```python
from build123d import *

# Parameters (mm, degrees)
EXTRUDE006_DEPTH = 2
EXTRUDE005_DEPTH = 2.25


with BuildPart() as extrude006:
    # Sketch006 → Extrude006 (new body)
    with BuildSketch(Plane.XZ):
        with BuildLine():
            ThreePointArc((16.9, 15.75), (15.9, 14.75), (16.9, 13.75))
            Line((16.9, 13.75), (23.5, 13.75))
            ThreePointArc((23.5, 13.75), (24.5, 14.75), (23.5, 15.75))
            Line((23.5, 15.75), (16.9, 15.75))
        make_face()
    extrude(amount=EXTRUDE006_DEPTH)


with BuildPart() as extrude006_1:
    # Extrude006 placement: moved
    add(extrude006.part.moved(Location((0, 4, 0))))


with BuildPart() as obj1:
    # Sketch005 → Extrude005 (new body)
    with BuildSketch(Plane.XZ):
        with BuildLine():
            ThreePointArc((16.9, 17.35), (15.9, 16.35), (16.9, 15.35))
            Line((16.9, 15.35), (23.5, 15.35))
            ThreePointArc((23.5, 15.35), (24.5, 16.35), (23.5, 17.35))
            Line((23.5, 17.35), (16.9, 17.35))
        make_face()
    extrude(amount=EXTRUDE005_DEPTH)


with BuildPart() as obj1_1:
    # Extrude005 placement: moved
    add(obj1.part.moved(Location((0, 2, 0))))

    # Fusion008: union Extrude006
    add(extrude006_1.part)


with BuildPart() as obj1_2:
    # Fusion008 placement: moved
    add(obj1_1.part.moved(Location((0, 0.25, 0))))


solid = obj1_2.part
```
For this review, take the finished solid that the model builds, in its own axes (mm). A direction names the side the tool comes from. Coordinates: 2 decimals unless noted, no trailing zeros. Write each loop counter-clockwise with the first axis right and the second up, starting at its lowest first coordinate (ties: lowest second). Pieces come first, ordered by that corner, then holes.
(1) For pin 1 Ø1 at (x, y) = (19.5, 3.5) entering from +Z; pin 2 Ø2 at (y, z) = (1, 15) entering from +X; pin 3 Ø1.1 at (x, y) = (21.5, 1) entering from -Z, all flat-tipped, find the tip position at first contact; note any pin that passes through.
(2) Add section A-A on x = 17. Give the boundary of the cut face in (y, z).
(3) Wall thickness on probe 1 along Z at (x, y) = (22.25, 1.1); probe 2 along Z at (x, y) = (23.25, 3.35); probe 3 along Y at (x, z) = (19.25, 16.8): over which ranges is each line inside the solid? List them lowest first.
(4) Tool access review of faces 1 (the face through (20, 1, 15.35)), 2 (the face through (20, 3, 15.75)), 3 (the face through (24.5, 1.1, 16.3)): name each direction out of +Z, -Z, +X, -X, +Y, -Y from which nothing blocks a thin tool from reaching the whole face with its end or side.
(5) Add section B-B on z = 16.35. Give the boundary of the cut face in (x, y).
(6) Add section C-C on y = 1.1. Give the boundary of the cut face in (x, z), then the cut area to 3 significant figures.
Answer sheet:
1. pin 1: stops at z = 15.75
1. pin 2: stops at x = 24.44
1. pin 3: stops at z = 15.35
2. outline: (0, 15.35) - (2.25, 15.35) - (2.25, 13.75) - (4.25, 13.75) - (4.25, 15.75) - (2.25, 15.75) - (2.25, 17.35) - (0, 17.35) - close
3. probe 1: z = 15.35 to 17.35
3. probe 2: z = 13.75 to 15.75
3. probe 3: y = 0 to 2.25
4. face 1: -Z, +X, -X, -Y
4. face 2: +Z, +X, -X, +Y
4. face 3: +X, -Y
5. outline: (15.9, 0) - (24.5, 0) - (24.5, 2.25) - (15.9, 2.25) - close
6. outline: (16.9, 15.35) - (23.5, 15.35) arc R1 ccw to (23.5, 17.35) - (16.9, 17.35) arc R1 ccw to start
6. area: 16.3 mm2
